Check sheet for the modelled part. Datum: model origin and axes. Units: mm. A direction names the side the tool comes from. Coordinates: 2 decimals unless noted, no trailing zeros. Write each loop counter-clockwise with the first axis right and the second up, starting at its lowest first coordinate (ties: lowest second). Pieces come first, ordered by that corner, then holes. Notation, with made-up numbers: M 42,2 L 54,2 A24 ccw 54,21 Z; hole C 31,24.5 d3. An arc over 180 degrees is marked long. Answer as CSV lines item,"result".
from build123d import *

# Parameters (mm, degrees)
F0_W     = 358.5
F0_H     = 139
F1_DEPTH = 10.575
F3_DEPTH = 358.501
F4_R     = 8.125
F4_R_2   = 6.25
F4_R_3   = 22.5
F5_DEPTH = 21.151


with BuildPart() as f1:
    # F0 (on Top) → F1 (new body, symmetric)
    with BuildSketch(Plane.XY):
        Rectangle(F0_W, F0_H)
    extrude(amount=F1_DEPTH, both=True)

    # F2 (on face) → F3 (cut, through all)
    with BuildSketch(Plane.YZ.offset(179.25)):
        Polygon((69.5, -8.975), (62.15, -8.975), (54.5, -1.325), (45.25, -10.575), (69.5, -10.575), align=None)
    extrude(amount=-F3_DEPTH, mode=Mode.SUBTRACT)

    # F4 (on face) → F5 (cut, through all)
    with BuildSketch(Plane(origin=(0, 0, -10.575), x_dir=(1, 0, 0), z_dir=(0, 0, -1))):
        with Locations((148.25, -0.47)):
            Circle(F4_R)
        with Locations((-146.45, -0.47)):
            Circle(F4_R)
        with Locations((-62.25, 24.03)):
            Circle(F4_R_2)
        with Locations((9.25, -24.57)):
            Circle(F4_R_3)
    extrude(amount=-F5_DEPTH, mode=Mode.SUBTRACT)


solid = f1.part
1) Section check A-A, the plane y = 24.57. Record the boundary of the cut face in (x, z) (3 decimals).
Answer key:
outline,"M -179.25,-10.575 L -13.25,-10.575 L -13.25,10.575 L -179.25,10.575 Z; M 31.75,-10.575 L 179.25,-10.575 L 179.25,10.575 L 31.75,10.575 Z"
2) Depth check by flat-ended pin: P1, Ø3.5, axis at x = 89, y = 65.5, coming from the -Z side (3 decimals); P2, Ø14.5, axis at x = -62.25, y = -24.03, coming from the -Z side (3 decimals). Enter the tip coordinate at first touch or a pass-through.
Answer key:
P1,"stops at z = -8.975"
P2,"stops at z = -10.575"
3) Section check B-B, the plane x = -146.45. Record the boundary of the cut face in (y, z) (3 decimals), plus the area to 3 significant figures.
Answer key:
outline,"M -69.5,-10.575 L -7.655,-10.575 L -7.655,10.575 L -69.5,10.575 Z; M 8.595,-10.575 L 45.25,-10.575 L 54.5,-1.325 L 62.15,-8.975 L 69.5,-8.975 L 69.5,10.575 L 8.595,10.575 Z"
area,"2,500 mm2"
4) Thickness scan on line 1 along X through (y, z) = (0.47, 2.25) (3 decimals); line 2 along X through (y, z) = (24.57, -1.5); line 3 along Y through (x, z) = (-146.45, 5) (3 decimals). Record the ranges inside material, lowest first.
Answer key:
line 1,"x = -179.25 to -154.575, -138.325 to 140.125, 156.375 to 179.25"
line 2,"x = -179.25 to -13.25, 31.75 to 179.25"
line 3,"y = -69.5 to -7.655, 8.595 to 69.5"
5) Tool access check on faces 1 (the face through (2.51, 49.94, -5.885)), 2 (the face through (-3, -69.5, 0)), 3 (the face through (3, 66, -8.975)). Record the directions out of +Z, -Z, +X, -X, +Y, -Y that give a thin tool (end or side, any length) a straight path to the whole face; none if there is none.
Answer key:
face 1,"-Z, +X, -X"
face 2,"+Z, -Z, +X, -X, -Y"
face 3,"-Z, +X, -X, +Y"
6) Section check D-D, the plane x = -100.5. Record the boundary of the cut face in (y, z) (3 decimals), plus the area to 3 significant figures.
Answer key:
outline,"M -69.5,-10.575 L 45.25,-10.575 L 54.5,-1.325 L 62.15,-8.975 L 69.5,-8.975 L 69.5,10.575 L -69.5,10.575 Z"
area,"2,840 mm2"
7) Mould release check, pull along X, two halves, no side actions. Record for faces 4 (the face through (-56.477, -21.636, -0.148)), 5 (the face through (179.25, -1, 0)), 6 (the face through (-3, 1, 10.575)), 7 (the face through (-179.25, -1, 0)): pulls with the +X half, pulls with the -X half, needs draft (parallel to the pull), parting line crosses it, or undercut.
Answer key:
face 4,"undercut"
face 5,"pulls with the +X half"
face 6,"needs draft"
face 7,"pulls with the -X half"
8) Section check C-C, the plane z = 2.25. Record the boundary of the cut face in (x, y) (3 decimals).
Answer key:
outline,"M -179.25,-69.5 L 179.25,-69.5 L 179.25,69.5 L -179.25,69.5 Z; hole C -146.45,0.47 d16.25; hole C -62.25,-24.03 d12.5; hole C 9.25,24.57 d45; hole C 148.25,0.47 d16.25"
